Autodesk Inventor part; units mm, degrees
ref_plane "Work Plane1" through (29, 0, 0) normal (0, -1, 0) x (1, 0, 0)
ref_plane "YZ Plane" through (0, 0, 0) normal (1, 0, 0) x (0, 1, 0)
ref_plane "XZ Plane" through (0, 0, 0) normal (0, 1, 0) x (-1, 0, 0)
sketch "Szkic1" plane through (0, 0, 0) normal (0, 0, 1) x (1, 0, 0)
  line L0 (-1.1667, 0) -> (16, 0)
  line L1 (16, 0) -> (16, 2.5)
  line L2 (16, 2.5) -> (2.4, 2.5)
  line L3 (2.4, 2.5) -> (1.9091, 2.5)
  line L4 (1.9091, 2.5) -> (0, 2.5)
  line L5 (0, 2.5) -> (0, 4.25)
  line L6 (0, 4.25) -> (-5, 4.25)
  line L7 (-5, 4.25) -> (-5, 2.3094)
  line L8 (-5, 2.3094) -> (-2.5, 2.3094)
  line L9 (-2.5, 2.3094) -> (-1.1667, 0)
  line L10 (-9.2, 0) -> (20.2, 0)
  line L11 (0, -0.85) -> (0, 5.1)
  line L12 (2.4, 2.5) -> (0, 2.5) construction
  dimension "d1" = 13.6
  dimension "d2" = 0.4909
  dimension "d3" = 5
  dimension "d4" = 2.5
  dimension "d5" = 60
  dimension "d6" = 5
  dimension "d7" = 5
  dimension "d8" = 4.6188
  dimension "d9" = 8.5
  dimension "d26" = 16
revolve "Bryła" add sketch "Szkic1" angle 360 about axis through (-1.1667, 0, 0) along (1, 0, 0)
sketch "Szkic2" plane through (-5, 0, 0) normal (-1, 0, 0) x (0, 0, 1)
  circle A0 centre (0, 0) radius 2.3094
  line L0 (0, -5.95) -> (0, 5.95)
  line L1 (-5.95, 0) -> (5.95, 0)
  line L2 (2.3094, 0) -> (1.1547, -2)
  line L3 (1.1547, -2) -> (-1.1547, -2)
  line L4 (-1.1547, -2) -> (-2.3094, 0)
  line L5 (-2.3094, 0) -> (-1.1547, 2)
  line L6 (-1.1547, 2) -> (1.1547, 2)
  line L7 (1.1547, 2) -> (2.3094, 0)
extrude "Szczelina" add sketch "Szkic2" against normal up to next contours L7 A0 | A0 L2 | L6 L0 A0 | A0 L0 L3 | L0 L6 A0 | A0 L3 L0 | L4 A0 | A0 L5
fillet "Zaokrąglenie1" radius 0.5 1 edges at (-5, -4.25, 0)
thread "Gwint"
chamfer "Faza1" distance 0.4908 distance2 0.4908 1 edges at (16, -2.5, 0) measured on face at (16, -1.1374, -1.1324)
ref_plane "Work Plane1" through (29, 0, 0) normal (0, -1, 0) x (1, 0, 0)
fillet "Fillet2" radius 0.1 1 edges at (0, -2.5, 0)
equation "\"d1\" = GEL"
equation "\"d3\" = KOH"
equation "\"d4\" = INTI"
equation "\"d6\" = GD"
equation "\"d7\" = BDM"
equation "\"d8\" = 1.1547 * SW"
equation "\"d9\" = KOD"
equation "\"d26\" = NLG"
equation "\"d30\" = R"
equation "\"d17\" = RR"
equation "\"d13\" = GEL"
equation "\"d15\" = -0.5 * SPD + 0.5 * GD"
equation "\"d16\" = GUL"
equation "\"GD\" = 5"
equation "\"NLG\" = 16"
equation "\"GEL\" = 13.6"
equation "\"KOD\" = 8.5"
equation "\"KOH\" = 5"
equation "\"INTI\" = 2.5"
equation "\"GAL\" = 0.61345 * PTC"
equation "\"GUL\" = 0.61345 * PTC"
equation "\"BDM\" = NND"
equation "\"SW\" = 4"
equation "\"RR\" = 0.5"
equation "\"SPD\" = NND - 1.2269 * PTC"
equation "\"R\" = 0.1"
equation "\"TOA\" = 30deg"
equation "\"GD1\" = THREADDIA - 1.2269 * PTC"
equation "\"THREADDIA\" = 5"
equation "\"FAWI\" = 45deg"
equation "\"PTC\" = 0.8"
equation "\"NND\" = 5"
equation "\"E0\" = 1.155 * SW"
properties part number "ISO 4762  - M5 x 16" material "Stal nierdzewna 440C"
Check sheet for the modelled part. Datum: model origin and axes. Units: mm. A direction names the side the tool comes from. Coordinates: 2 decimals unless noted, no trailing zeros. Write each loop counter-clockwise with the first axis right and the second up, starting at its lowest first coordinate (ties: lowest second). Pieces come first, ordered by that corner, then holes. Notation, with made-up numbers: M 56,34 L 91,34 A8 ccw 91,46 Z; hole C 25.25,86.5 d10. An arc over 180 degrees is marked long. Answer as CSV lines item,"result".
Q1. Mould release check, pull along Z, two halves, no side actions. Record for faces 1 (the face through (7.7, -0.54, 2.44)), 2 (the face through (16, 0, 0)), 3 (the face through (-3.679, -1.014, -1.724)): released by +Z, released by -Z, zero draft, split by the parting line, or undercut.
Check result:
face 1,"split by the parting line"
face 2,"zero draft"
face 3,"undercut"
Q2. Go/stop test with flat-tipped pins: pin 1 (1 mm diameter, centred on x = 8.5, z = 2, fed in from +Y); pin 2 (5 mm diameter, centred on x = 12.5, z = 1.5, fed in from -Y); pin 3 (1.5 mm diameter, centred on x = 13, z = 0, fed in from +Y). Record where each tip stops, or that it passes through.
Check result:
pin 1,"y = 2"
pin 2,"y = -2.5"
pin 3,"y = 2.5"
Q3. Material ranges on probe 1 along X at (y, z) = (3, 1); probe 2 along X at (y, z) = (0, -2); probe 3 along Y at (x, z) = (-2, -2), recorded low to high. Write a range as from..to.
Check result:
probe 1,"-5..0"
probe 2,"-2.32..16"
probe 3,"-3.75..3.75"
Q4. Cross-section at A-A (x = 0.75). Record the boundary of the cut face in (y, z), then the cut area to 3 significant figures.
Check result:
outline,"C 0,0 d5"
area,"19.6 mm^2"
Q5. Set-up check for faces 4 (the face through (0, 2, 2)), 5 (the face through (-4, 2, 0)), 6 (the face through (-5, -2, 2)): record each of +Z, -Z, +X, -X, +Y, -Y from which the full face is reachable in a straight line by a thin tool's end or side.
Check result:
face 4,"+X"
face 5,"-X"
face 6,"+Z, -Z, -X, +Y, -Y"
